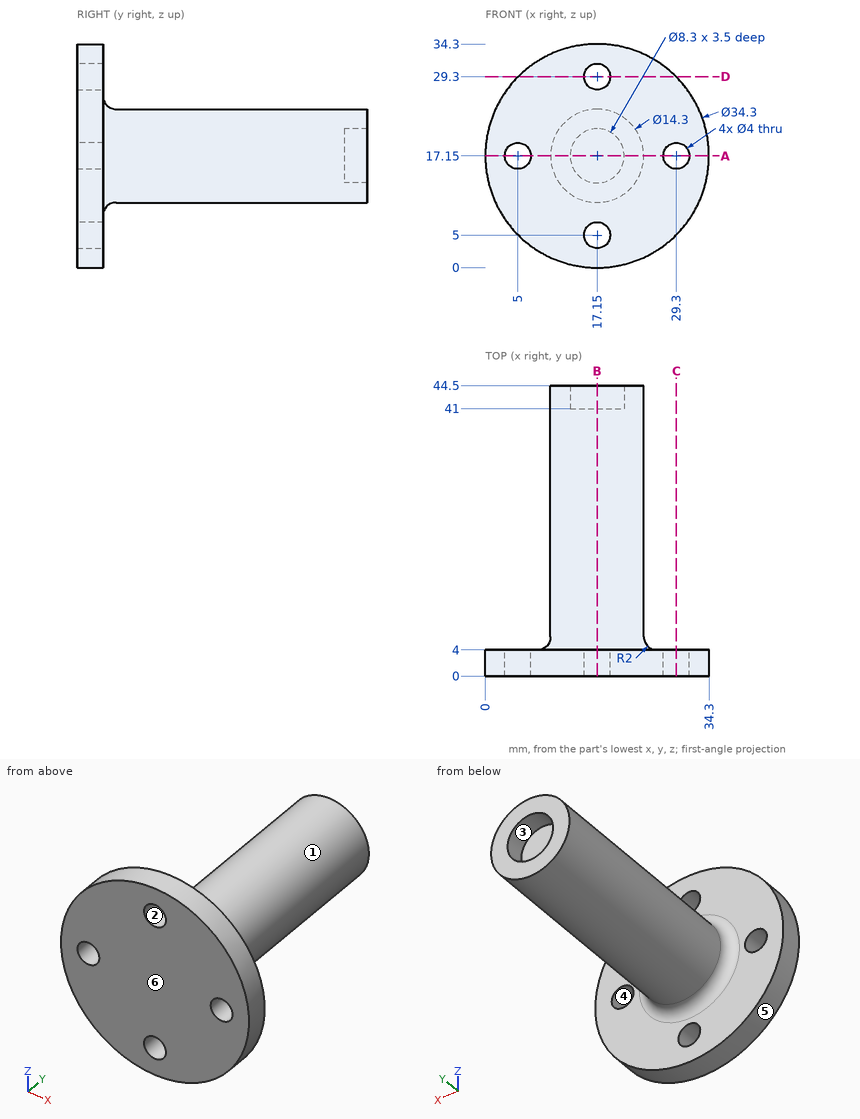
Input: dimensioned drawing with shaded views. Units: mm. Origin: part minimum x, y, z. A direction names the side the tool comes from. Coordinates: 2 decimals unless noted, no trailing zeros. Write each loop counter-clockwise with the first axis right and the second up, starting at its lowest first coordinate (ties: lowest second). Pieces come first, ordered by that corner, then holes. Notation, with made-up numbers: M 37.5,21 L 66.5,21 A24 cw 66.5,51 Z; hole C 69,30.5 d5. An arc over 180 degrees is marked long. Answer as a JSON object with one key per item and string values. Group by question number.
(1) Section A-A on z = 17.15. Output: boundary loops of the cut face in (x, y), plus the area to 3 significant figures.
(2) Contact query for flat-ended pins moving along their axis: P1, Ø2, axis at y = 22.5, z = 14.5, coming from the -X side; P2, Ø1.5, axis at y = 36, z = 20, coming from the +X side; P3, Ø5, axis at y = 11.5, z = 15, coming from the -X side. Output: stop coordinate, or through.
(3) Section D-D on z = 29.3. Output: boundary loops of the cut face in (x, y), plus the area to 3 significant figures.
(4) Ray query, line 1 along Z through (x, y) = (17, 2); line 2 along X through (y, z) = (2.55, 17.15); line 3 along X through (y, z) = (43.85, 17.15). Return the intervals inside material, ascending. Write a range as [from, to].
(5) Section B-B on x = 17.15. Output: boundary loops of the cut face in (y, z).
(6) Section C-C on x = 29.3. Output: boundary loops of the cut face in (y, z), plus the area to 3 significant figures.
(7) Set-up query: the marked faces 1 and 2. Return all of +Z, -Z, +X, -X, +Y, -Y with unobstructed straight access to the full face (end or side cutting, diameter ignored); none if empty.
(8) Mould query, pull axis Z, two halves, no side actions, for the marked faces 3, 4, 5 and 6. Classes: pulls with the +Z half, pulls with the -Z half, needs draft (parallel to the pull), parting line crosses it, or undercut.
Result set:
{
 "1": {"outline": "M 0,0 L 3,0 L 3,4 L 0,4 Z; M 7,0 L 27.3,0 L 27.3,4 L 26.3,4 A2 cw 24.3,6 L 24.3,44.5 L 21.3,44.5 L 21.3,41 L 13,41 L 13,44.5 L 10,44.5 L 10,6 A2 cw 8,4 L 7,4 Z; M 31.3,0 L 34.3,0 L 34.3,4 L 31.3,4 Z", "area": "657 mm2"},
 "2": {"P1": "stops at x = 10.19", "P2": "stops at x = 23.98", "P3": "stops at x = 10"},
 "3": {"outline": "M 5.05,0 L 15.15,0 L 15.15,4 L 5.05,4 Z; M 19.15,0 L 29.25,0 L 29.25,4 L 19.15,4 Z", "area": "80.8 mm2"},
 "4": {"line 1": "z = [0, 3.01], [6.99, 27.31], [31.29, 34.3]", "line 2": "x = [0, 3], [7, 27.3], [31.3, 34.3]", "line 3": "x = [10, 13], [21.3, 24.3]"},
 "5": {"outline": "M 0,0 L 4,0 L 4,3 L 0,3 Z; M 0,7 L 4,7 L 4,8 A2 cw 6,10 L 44.5,10 L 44.5,13 L 41,13 L 41,21.3 L 44.5,21.3 L 44.5,24.3 L 6,24.3 A2 cw 4,26.3 L 4,27.3 L 0,27.3 Z; M 0,31.3 L 4,31.3 L 4,34.3 L 0,34.3 Z"},
 "6": {"outline": "M 0,5.05 L 4,5.05 L 4,15.15 L 0,15.15 Z; M 0,19.15 L 4,19.15 L 4,29.25 L 0,29.25 Z", "area": "80.8 mm2"},
 "7": {"face 1": "+Y", "face 2": "+Y, -Y"},
 "8": {"face 3": "undercut", "face 4": "undercut", "face 5": "parting line crosses it", "face 6": "needs draft"}
}
